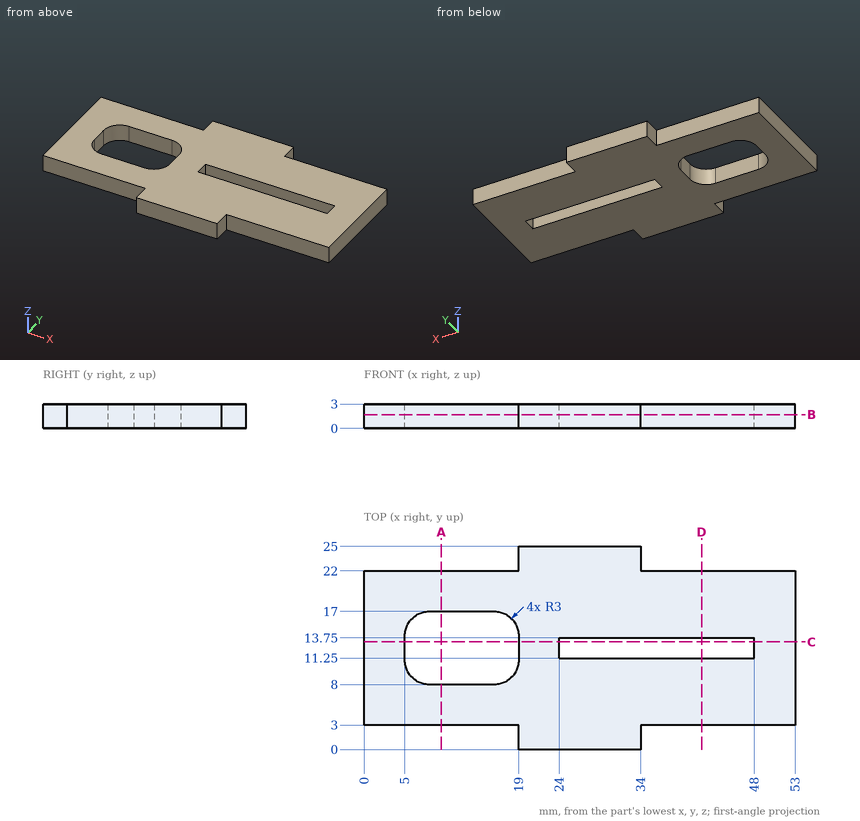
Check sheet for the drawn part. Datum: minimum x, y, z corner. Units: mm. Round coordinates to 2 decimals unless told otherwise and drop trailing zeros. Order: outer loops, then holes, each group sorted by start corner. A loop starts at its lowest first (then second) coordinate and runs counter-clockwise, first axis right, second up. Notation, with made-up numbers: (57.25, 42) -> (98.25, 42) arc R19 cw to (98.25, 49) -> close; hole circle Ø3 at (-3.75, 29.5). An arc over 180 degrees is marked (long way). Put each result on its own line as item: value. Start each with the question number.
(1) Depth check by flat-ended pin: pin 1 Ø1.5 at (y, z) = (1.5, 2) entering from +X; pin 2 Ø1.5 at (x, z) = (5, 1.5) entering from +Y; pin 3 Ø1.5 at (x, z) = (47, 1) entering from -Y. Enter the tip coordinate at first touch or a pass-through.
(2) Section check A-A (x = 9.5). Enter the section's corners in (y, z).
(3) Section check C-C (y = 13.25). Enter the section's corners in (x, z).
(4) Section check B-B (z = 1.7). Enter the section's corners in (x, y), then the cut area to 3 significant figures.
(5) Material ranges on line 1 along X through (y, z) = (13.5, 1.8); line 2 along X through (y, z) = (14.25, 0.6); line 3 along Y through (x, z) = (46.5, 2.05), recorded low to high.
(6) Section check D-D (x = 41.5). Enter the section's corners in (y, z).
Completed:
1. pin 1: stops at x = 34
1. pin 2: stops at y = 22
1. pin 3: stops at y = 3
2. outline: (3, 0) -> (8, 0) -> (8, 3) -> (3, 3) -> close; (17, 0) -> (22, 0) -> (22, 3) -> (17, 3) -> close
3. outline: (0, 0) -> (5, 0) -> (5, 3) -> (0, 3) -> close; (19, 0) -> (24, 0) -> (24, 3) -> (19, 3) -> close; (48, 0) -> (53, 0) -> (53, 3) -> (48, 3) -> close
4. outline: (0, 3) -> (19, 3) -> (19, 0) -> (34, 0) -> (34, 3) -> (53, 3) -> (53, 22) -> (34, 22) -> (34, 25) -> (19, 25) -> (19, 22) -> (0, 22) -> close; hole (5, 11) arc R3 ccw to (8, 8) -> (16, 8) arc R3 ccw to (19, 11) -> (19, 14) arc R3 ccw to (16, 17) -> (8, 17) arc R3 ccw to (5, 14) -> close; hole (24, 11.25) -> (48, 11.25) -> (48, 13.75) -> (24, 13.75) -> close
4. area: 919 mm2
5. line 1: x = 0 to 5, 19 to 24, 48 to 53
5. line 2: x = 0 to 5.01, 18.99 to 53
5. line 3: y = 3 to 11.25, 13.75 to 22
6. outline: (3, 0) -> (11.25, 0) -> (11.25, 3) -> (3, 3) -> close; (13.75, 0) -> (22, 0) -> (22, 3) -> (13.75, 3) -> close
